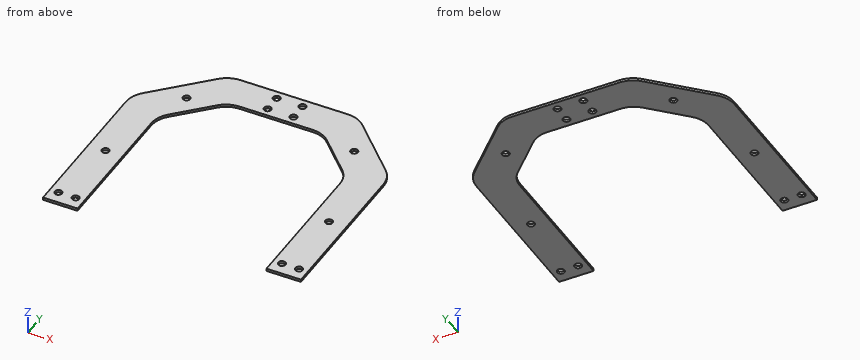
```python
from build123d import *

# Parameters (mm, degrees)
SALIENTE_EXTRUIR1_DEPTH      = 3
TALADRO_DE_MARGEN_PARA_M81_D = 8.4


with BuildPart() as part:
    # Croquis1 → Saliente-Extruir1 (new body)
    with BuildSketch(Plane.XY):
        with BuildLine():
            Line((-63.536796564, 221.213203436), (-100.713203436, 184.036796564))
            ThreePointArc((-100.713203436, 184.036796564), (-107.216385975, 174.3040961), (-109.5, 162.823593129))
            Line((-109.5, 162.823593129), (-109.5, 0))
            Line((-109.5, 0), (-149.5, 0))
            Line((-149.5, 0), (-149.5, 182.823593129))
            ThreePointArc((-149.5, 182.823593129), (-147.216385975, 194.3040961), (-140.713203436, 204.036796564))
            Line((-140.713203436, 204.036796564), (-83.536796564, 261.213203436))
            ThreePointArc((-83.536796564, 261.213203436), (-73.8040961, 267.716385975), (-62.323593129, 270))
            Line((-62.323593129, 270), (62.323593129, 270))
            ThreePointArc((62.323593129, 270), (73.8040961, 267.716385975), (83.536796564, 261.213203436))
            Line((83.536796564, 261.213203436), (140.713203436, 204.036796564))
            ThreePointArc((140.713203436, 204.036796564), (147.216385975, 194.3040961), (149.5, 182.823593129))
            Line((149.5, 182.823593129), (149.5, 0))
            Line((149.5, 0), (109.5, 0))
            Line((109.5, 0), (109.5, 162.823593129))
            ThreePointArc((109.5, 162.823593129), (107.216385975, 174.3040961), (100.713203436, 184.036796564))
            Line((100.713203436, 184.036796564), (63.536796564, 221.213203436))
            ThreePointArc((63.536796564, 221.213203436), (53.8040961, 227.716385975), (42.323593129, 230))
            Line((42.323593129, 230), (-42.323593129, 230))
            ThreePointArc((-42.323593129, 230), (-53.8040961, 227.716385975), (-63.536796564, 221.213203436))
        make_face()
    extrude(amount=SALIENTE_EXTRUIR1_DEPTH)

    # Taladro de margen para M81 (through all)
    with Locations(Plane.XY.offset(3)):
        with Locations((-119.5, 15), (-139.5, 15), (0, 15), (139.5, 15), (-15, 260), (-15, 240), (15, 240), (15, 260), (-129.5, 100.125), (-97.125, 217.625), (129.5, 100.125), (97.125, 217.625), (119.5, 15)):
            Hole(TALADRO_DE_MARGEN_PARA_M81_D / 2)


solid = part.part
```
Verification items for the finished model (mm, model axes). Coordinates: 2 decimals unless noted, no trailing zeros. Order: outer loops, then holes, each group sorted by start corner. A loop starts at its lowest first (then second) coordinate and runs counter-clockwise, first axis right, second up. Notation, with made-up numbers: (53.25, 8.25) -> (107.25, 8.25) arc R20 ccw to (107.25, 25.25) -> close; hole circle Ø8 at (8, 63). An arc over 180 degrees is marked (long way). Put each result on its own line as item: value. Start each with the question number.
1) Cross-section at B-B (x = 129.5). Enter the section's corners in (y, z) (3 decimals), plus the area to 3 significant figures.
2) Cross-section at C-C (x = -15). Enter the section's corners in (y, z).
3) Go/stop test with flat-tipped pins: pin 1 (7.5 mm diameter, centred on x = 15, y = 240, fed in from -Z); pin 2 (1.5 mm diameter, centred on x = 84.5, z = 1, fed in from -Y); pin 3 (1.5 mm diameter, centred on x = 14, z = 1, fed in from -Y); pin 4 (1 mm diameter, centred on x = 54.5, z = 0.5, fed in from -Y). Record where each tip stops, or that it passes through.
4) Material ranges on L1, parallel to Y at x = 15, z = 0.7; L2, parallel to X at y = 49, z = 1.15; L3, parallel to X at y = 101, z = 2.8, recorded low to high.
5) Cross-section at A-A (y = 139.5). Enter the section's corners in (x, z).
6) Cross-section at D-D (z = 0.75). State how many separate pieces and enclosed holes the cut face has, plus the area to 3 significant figures.
Geometry check:
1. outline: (0, 0) -> (95.925, 0) -> (95.925, 3) -> (0, 3) -> close; (104.325, 0) -> (215.25, 0) -> (215.25, 3) -> (104.325, 3) -> close
1. area: 621 mm^2
2. outline: (230, 0) -> (235.8, 0) -> (235.8, 3) -> (230, 3) -> close; (244.2, 0) -> (255.8, 0) -> (255.8, 3) -> (244.2, 3) -> close; (264.2, 0) -> (270, 0) -> (270, 3) -> (264.2, 3) -> close
3. pin 1: passes through
3. pin 2: stops at y = 199.5
3. pin 3: stops at y = 230
3. pin 4: stops at y = 227.19
4. L1: y = 230 to 235.8, 244.2 to 255.8, 264.2 to 270
4. L2: x = -149.5 to -109.5, 109.5 to 149.5
4. L3: x = -149.5 to -133.61, -125.39 to -109.5, 109.5 to 125.39, 133.61 to 149.5
5. outline: (-149.5, 0) -> (-109.5, 0) -> (-109.5, 3) -> (-149.5, 3) -> close; (109.5, 0) -> (149.5, 0) -> (149.5, 3) -> (109.5, 3) -> close
6. separate pieces: 1
6. enclosed holes: 12
6. area: 27,100 mm^2
